Job drawing, mm, ordinate dimensions from the low corner. One solid piece. Give positions to 0.01 mm unless a question says otherwise; leave off trailing zeros. Loops run counter-clockwise (first coordinate to the right, second up) from the corner with the lowest first, then second, coordinate; pieces in that order, holes last. Notation, with made-up numbers: M 88.5,-39 L 146.5,-39 A15 cw 146.5,-27 Z; hole C 36.5,73 d9. An arc over 180 degrees is marked long. Answer in a Markdown table with one row per item.
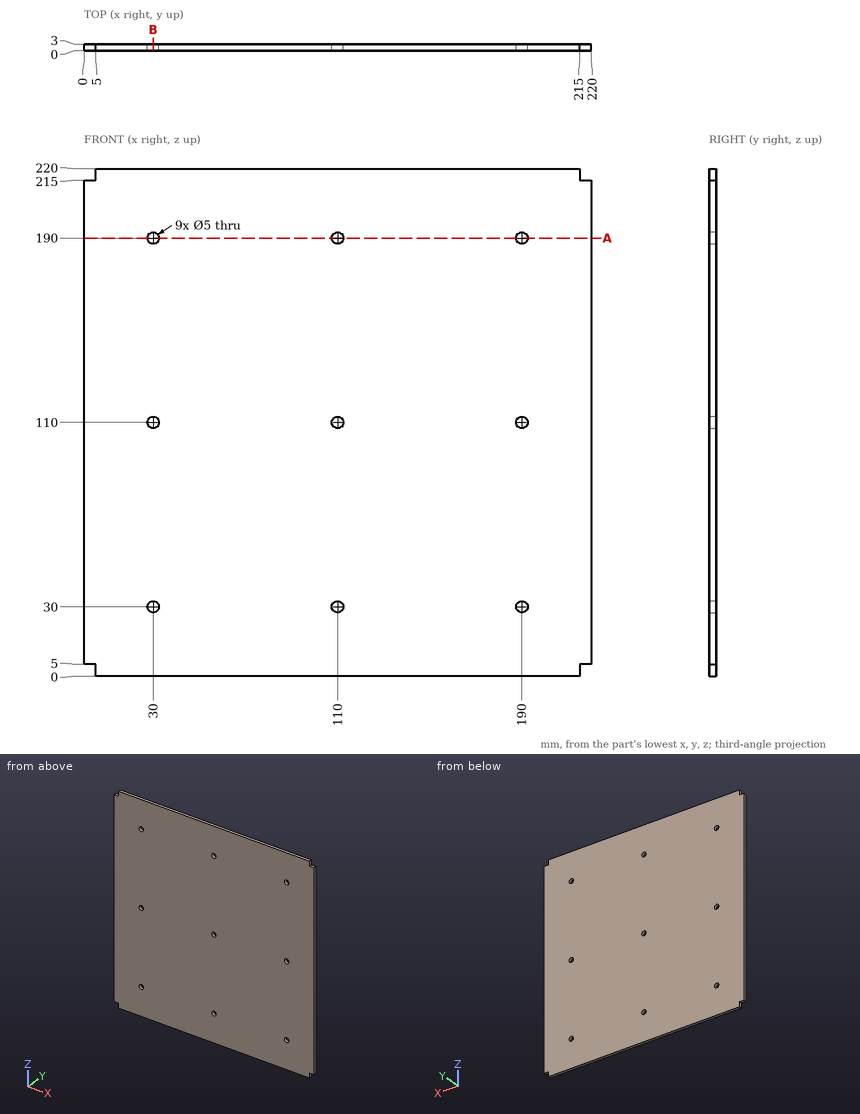
(1) Saw through at B-B (x = 30). Write the cut outline in (y, z).
Recorded:
| item | result |
|---|---|
| outline | M 0,0 L 3,0 L 3,27.5 L 0,27.5 Z; M 0,32.5 L 3,32.5 L 3,107.5 L 0,107.5 Z; M 0,112.5 L 3,112.5 L 3,187.5 L 0,187.5 Z; M 0,192.5 L 3,192.5 L 3,220 L 0,220 Z |
(2) Saw through at A-A (z = 190). Write the cut outline in (x, y).
Recorded:
| item | result |
|---|---|
| outline | M 0,0 L 27.5,0 L 27.5,3 L 0,3 Z; M 32.5,0 L 107.5,0 L 107.5,3 L 32.5,3 Z; M 112.5,0 L 187.5,0 L 187.5,3 L 112.5,3 Z; M 192.5,0 L 220,0 L 220,3 L 192.5,3 Z |
(3) Drill centre lines: line 1 along Z through (x, y) = (110, 1.5); line 2 along X through (y, z) = (0.2, 188). Where is each one in solid material? Low to high.
Recorded:
| item | result |
|---|---|
| line 1 | z = 0 to 27.5, 32.5 to 107.5, 112.5 to 187.5, 192.5 to 220 |
| line 2 | x = 0 to 28.5, 31.5 to 108.5, 111.5 to 188.5, 191.5 to 220 |
(4) Pin check, flat tips, straight feed: pin 1 Ø6.5 at (x, z) = (30, 190) entering from -Y; pin 2 Ø1.5 at (x, y) = (1.5, 2) entering from +Z; pin 3 Ø1.5 at (y, z) = (1, 216.5) entering from -X; pin 4 Ø1.5 at (y, z) = (2, 3.5) entering from +X. Stop position of each tip, or through.
Recorded:
| item | result |
|---|---|
| pin 1 | stops at y = 0 |
| pin 2 | stops at z = 215 |
| pin 3 | stops at x = 5 |
| pin 4 | stops at x = 215 |
